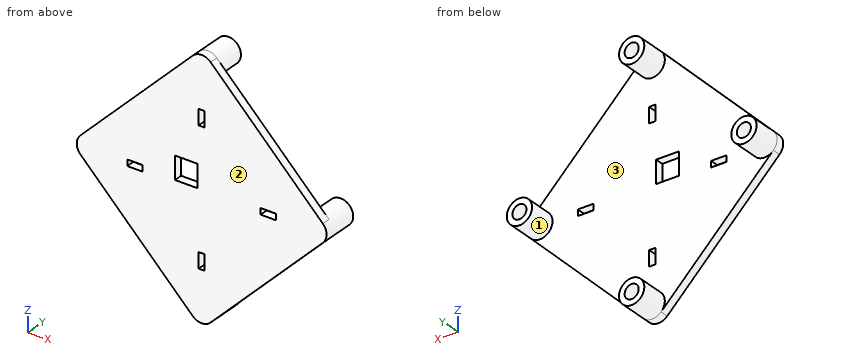
from build123d import *

# Parameters (mm, degrees)
SKETCH1_W           = 100
SKETCH1_H           = 100
BOSS_EXTRUDE1_DEPTH = 3
SKETCH2_R           = 4.5
SKETCH2_R_2         = 2.5
BOSS_EXTRUDE2_DEPTH = 10
SKETCH9_OUTSIDE_W   = 130.404
SKETCH9_OUTSIDE_H   = 130.404
CUT_EXTRUDE5_DEPTH  = 127
SKETCH11_W          = 8.1
SKETCH11_H          = 8.1
CUT_EXTRUDE6_DEPTH  = 127
SKETCH3_W           = 5.499999922
SKETCH3_H           = 2.2
SKETCH3_W_2         = 2.2
SKETCH3_H_2         = 5.499999922
CUT_EXTRUDE7_DEPTH  = 4


with BuildPart() as part:
    # Sketch1 → Boss-Extrude1 (new body)
    with BuildSketch(Plane(origin=(0, 0, 0), x_dir=(1, 0, 0), z_dir=(0, 1, 0))):
        Rectangle(SKETCH1_W, SKETCH1_H)
    extrude(amount=BOSS_EXTRUDE1_DEPTH)

    # Sketch2 → Boss-Extrude2 (add)
    with BuildSketch(Plane(origin=(0, 3, 0), x_dir=(1, 0, 0), z_dir=(0, 1, 0))):
        with Locations((0, 40)):
            Circle(SKETCH2_R)
        with Locations((0, 40)):
            Circle(SKETCH2_R_2, mode=Mode.SUBTRACT)
        with Locations((40, 0)):
            Circle(SKETCH2_R)
        with Locations((40, 0)):
            Circle(SKETCH2_R_2, mode=Mode.SUBTRACT)
        with Locations((0, -40)):
            Circle(SKETCH2_R)
        with Locations((0, -40)):
            Circle(SKETCH2_R_2, mode=Mode.SUBTRACT)
        with Locations((-40, 0)):
            Circle(SKETCH2_R)
        with Locations((-40, 0)):
            Circle(SKETCH2_R_2, mode=Mode.SUBTRACT)
    extrude(amount=BOSS_EXTRUDE2_DEPTH)

    # Sketch9 outside → Cut-Extrude5 (cut)
    with BuildSketch(Plane(origin=(0, 3, 0), x_dir=(1, 0, 0), z_dir=(0, 1, 0))):
        Rectangle(SKETCH9_OUTSIDE_W, SKETCH9_OUTSIDE_H)
        with BuildLine():
            Line((3.181980515, 43.181980515), (43.181980515, 3.181980515))
            ThreePointArc((43.181980515, 3.181980515), (44.5, 0), (43.181980515, -3.181980515))
            Line((43.181980515, -3.181980515), (3.181980515, -43.181980515))
            ThreePointArc((3.181980515, -43.181980515), (0, -44.5), (-3.181980515, -43.181980515))
            Line((-3.181980515, -43.181980515), (-43.181980515, -3.181980515))
            ThreePointArc((-43.181980515, -3.181980515), (-44.5, 0), (-43.181980515, 3.181980515))
            Line((-43.181980515, 3.181980515), (-3.181980515, 43.181980515))
            ThreePointArc((-3.181980515, 43.181980515), (0, 44.5), (3.181980515, 43.181980515))
        make_face(mode=Mode.SUBTRACT)
    extrude(amount=-CUT_EXTRUDE5_DEPTH, mode=Mode.SUBTRACT)

    # Sketch11 → Cut-Extrude6 (cut)
    with BuildSketch(Plane(origin=(0, 3, 0), x_dir=(1, 0, 0), z_dir=(0, 1, 0))):
        with Locations((-5.45, -3.85)):
            Rectangle(SKETCH11_W, SKETCH11_H)
    extrude(amount=-CUT_EXTRUDE6_DEPTH, mode=Mode.SUBTRACT)

    # Sketch3 → Cut-Extrude7 (cut, through all)
    with BuildSketch(Plane(origin=(0, 3, 0), x_dir=(1, 0, 0), z_dir=(0, 1, 0))):
        with Locations((23.749999998, 0.250000008)):
            Rectangle(SKETCH3_W, SKETCH3_H)
        with Locations((0, 24.000000006)):
            Rectangle(SKETCH3_W_2, SKETCH3_H_2)
        with Locations((0, -23.49999999)):
            Rectangle(SKETCH3_W_2, SKETCH3_H_2)
        with Locations((-23.749999998, 0.250000008)):
            Rectangle(SKETCH3_W, SKETCH3_H)
    extrude(amount=-CUT_EXTRUDE7_DEPTH, mode=Mode.SUBTRACT)


solid = part.part
Input: part model. Units: mm. Frame: model coordinates. Face numbers are marked on the shaded views. Coordinates: 2 decimals unless noted, no trailing zeros. Write each loop counter-clockwise with the first axis right and the second up, starting at its lowest first coordinate (ties: lowest second). Pieces come first, ordered by that corner, then holes. Notation, with made-up numbers: M 27.5,68.5 L 35.5,68.5 A30 cw 35.5,94.5 Z; hole C 81.5,-35.5 d10. An arc over 180 degrees is marked long. Answer as a JSON object with one key per item and string values. Group by question number.
(1) Mould query, pull axis Z, two halves, no side actions, for the marked faces 1, 2 and 3. Classes: pulls with the +Z half, pulls with the -Z half, needs draft (parallel to the pull), parting line crosses it, or undercut.
(2) Section C-C on z = -23. Output: boundary loops of the cut face in (x, y).
(3) Section B-B on x = 0. Output: boundary loops of the cut face in (y, z), plus the area to 3 significant figures.
(4) Section A-A on y = 7.25. Output: boundary loops of the cut face in (x, z).
(5) Section D-D on z = -40. Output: boundary loops of the cut face in (x, y), plus the area to 3 significant figures.
(6) Ray query, line 1 along Z through (x, y) = (0, 7.5); line 2 along Z through (x, y) = (40, 11.25). Return the intervals inside material, ascending. Write a range as [from, to].
(7) Contact query for flat-ended pins moving along their axis: P1, Ø1.1, axis at y = 1, z = -0.5, coming from the +X side; P2, Ø0.9, axis at y = 2, z = 4.5, coming from the +X side; P3, Ø2, axis at x = 5, y = 4, coming from the -Z side; P4, Ø0.7, axis at x = 0.5, y = 2, coming from the -Z side. Output: stop coordinate, or through.
Result set:
{
 "1": {"face 1": "parting line crosses it", "face 2": "needs draft", "face 3": "undercut"},
 "2": {"outline": "M -23.36,0 L -1.1,0 L -1.1,3 L -23.36,3 Z; M 1.1,0 L 23.36,0 L 23.36,3 L 1.1,3 Z"},
 "3": {"outline": "M 0,-44.5 L 13,-44.5 L 13,-42.5 L 3,-42.5 L 3,-37.5 L 13,-37.5 L 13,-35.5 L 3,-35.5 L 3,-26.75 L 0,-26.75 Z; M 0,-21.25 L 3,-21.25 L 3,20.75 L 0,20.75 Z; M 0,26.25 L 3,26.25 L 3,35.5 L 13,35.5 L 13,37.5 L 3,37.5 L 3,42.5 L 13,42.5 L 13,44.5 L 0,44.5 Z", "area": "314 mm2"},
 "4": {"outline": "C -40,0 d9; C 0,-40 d9; C 0,40 d9; C 40,0 d9; hole C -40,0 d5; hole C 0,-40 d5; hole C 0,40 d5; hole C 40,0 d5"},
 "5": {"outline": "M -6.36,0 L 6.36,0 L 6.36,3 L 4.5,3 L 4.5,13 L 2.5,13 L 2.5,3 L -2.5,3 L -2.5,13 L -4.5,13 L -4.5,3 L -6.36,3 Z", "area": "78.2 mm2"},
 "6": {"line 1": "z = [-44.5, -42.5], [-37.5, -35.5], [35.5, 37.5], [42.5, 44.5]", "line 2": "z = [-4.5, -2.5], [2.5, 4.5]"},
 "7": {"P1": "stops at x = 44.5", "P2": "stops at x = 42.31", "P3": "stops at z = -42.06", "P4": "stops at z = -44.5"}
}
